from build123d import *

# Parameters (mm, degrees)
BOSS_EXTRU_1_DEPTH            = 30
ENL_V_MAT_EXTRU_1_DEPTH       = 20
BOSS_EXTRU_3_DEPTH            = 340
ENL_V_MAT_EXTRU_2_DEPTH       = 710.357976131
ENL_V_START                   = -320
ENL_V_MAT_EXTRU_5_DEPTH       = 364
R_P_TITION_CIRCULAIRE13_COUNT = 6


with BuildPart() as part:
    # Esquisse1 → Boss.-Extru.1 (new body)
    with BuildSketch(Plane(origin=(0, 0, 0), x_dir=(1, 0, 0), z_dir=(0, 1, 0))):
        Polygon((312.198829019, 291.659432373), (-96.485063179, 416.201833149), (-408.683892198, 124.542400776), (-312.198829019, -291.659432373), (96.485063179, -416.201833149), (408.683892198, -124.542400776), align=None)
    extrude(amount=BOSS_EXTRU_1_DEPTH)

    # Esquisse2 → Enlèv. mat.-Extru.1 (cut)
    with BuildSketch(Plane(origin=(0, 30, 0), x_dir=(1, 0, 0), z_dir=(0, 1, 0))):
        Polygon((403.161136898, -122.85939536), (307.979925924, 287.718088693), (-95.181210974, 410.577484053), (-403.161136898, 122.85939536), (-307.979925924, -287.718088693), (95.181210974, -410.577484053), align=None)
    extrude(amount=-ENL_V_MAT_EXTRU_1_DEPTH, mode=Mode.SUBTRACT)

    # Esquisse5 → Boss.-Extru.3 (add)
    with BuildSketch(Plane(origin=(0, 10, 0), x_dir=(1, 0, 0), z_dir=(0, 1, 0))):
        Polygon((83.204563714, -358.91453872), (43.518265641, -422.554131312), (107.157858233, -462.240429385), (146.844156306, -398.600836793), align=None)
    boss_extru_3 = extrude(amount=BOSS_EXTRU_3_DEPTH)

    # Esquisse6 → Enlèv. mat.-Extru.2 (cut, through all)
    with BuildSketch(Plane(origin=(0, 350, 0), x_dir=(1, 0, 0), z_dir=(0, 1, 0))):
        Polygon((55.305373646, -403.65272736), (96.485063179, -416.201833149), (127.942752354, -386.813728788), (146.844156306, -398.600836793), (107.157858233, -462.240429385), (43.518265641, -422.554131312), align=None)
    enl_v_mat_extru_2 = extrude(amount=-ENL_V_MAT_EXTRU_2_DEPTH, mode=Mode.SUBTRACT)

    # Esquisse7 → Enlèv. mat.-Extru.5 (cut)
    with BuildSketch(Plane(origin=(0, 350, 0), x_dir=(1, 0, 0), z_dir=(0, 1, 0)).offset(ENL_V_START)):
        Polygon((58.044458918, -399.260423737), (55.305373646, -403.65272736), (96.485063179, -416.201833149), (127.942752354, -386.813728788), (123.550448731, -384.074643516), (95.181210974, -410.577484053), align=None)
    enl_v_mat_extru_5 = extrude(amount=ENL_V_MAT_EXTRU_5_DEPTH, mode=Mode.SUBTRACT)

    # Répétition circulaire13: Boss.-Extru.3, Enlèv. mat.-Extru.2, Enlèv. mat.-Extru.5 ×6 about axis
    r_p_tition_circulaire13_axis = Axis((0, 0, 0), (0, 1, 0))
    add([boss_extru_3.rotate(r_p_tition_circulaire13_axis, i * 360 / R_P_TITION_CIRCULAIRE13_COUNT) for i in range(1, R_P_TITION_CIRCULAIRE13_COUNT)])
    add([enl_v_mat_extru_2.rotate(r_p_tition_circulaire13_axis, i * 360 / R_P_TITION_CIRCULAIRE13_COUNT) for i in range(1, R_P_TITION_CIRCULAIRE13_COUNT)], mode=Mode.SUBTRACT)
    add([enl_v_mat_extru_5.rotate(r_p_tition_circulaire13_axis, i * 360 / R_P_TITION_CIRCULAIRE13_COUNT) for i in range(1, R_P_TITION_CIRCULAIRE13_COUNT)], mode=Mode.SUBTRACT)


solid = part.part
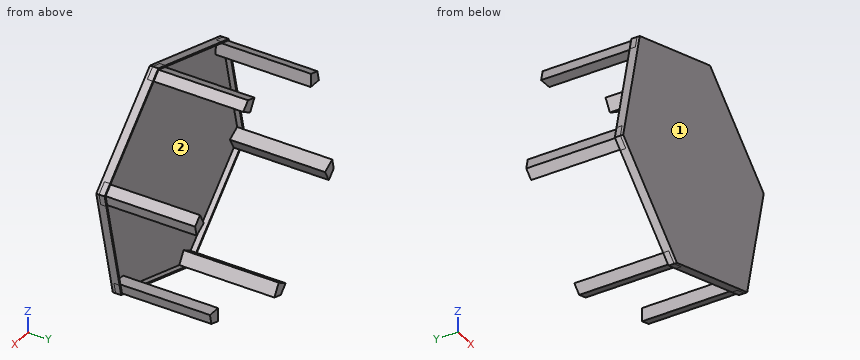
Read the model definition and answer for the solid it produces. Units are mm, in the model's axes. Face numbers are marked on the shaded views. Coordinates: 2 decimals unless noted, no trailing zeros. Write each loop counter-clockwise with the first axis right and the second up, starting at its lowest first coordinate (ties: lowest second). Pieces come first, ordered by that corner, then holes. Notation, with made-up numbers: M -11,39.5 L 30,39.5 A20 cw 30,72.5 Z; hole C 22.5,-33 d11. An arc over 180 degrees is marked long. Use a Markdown table: item, result.
Q1. Determine the mould class of the marked faces 1 and 2 for opening direction Z: released by +Z, released by -Z, zero draft, split by the parting line, or undercut.
Answer block:
| item | result |
|---|---|
| face 1 | zero draft |
| face 2 | undercut |
Q2. Each of these flat-tipped pins is pushed along its axis until it touches: pin 1 Ø2 at (x, z) = (135.5, 202.5) entering from -Y; pin 2 Ø1.5 at (x, y) = (291.5, 215.5) entering from -Z; pin 3 Ø8 at (x, y) = (76.5, 265.5) entering from +Z; pin 4 Ø4 at (x, y) = (-287, 246) entering from +Z. Where does it stop, or does it pass through?
Answer block:
| item | result |
|---|---|
| pin 1 | stops at y = 0 |
| pin 2 | stops at z = -292.97 |
| pin 3 | stops at z = 406.1 |
| pin 4 | stops at z = 294.72 |
Q3. The part is cut by section C-C, the plane x = 37. Write down the section's boundary in (y, z), then the cut area to 3 significant figures.
Answer block:
| item | result |
|---|---|
| outline | M 0,-375.52 L 30,-375.52 L 30,-370.3 L 10,-370.3 L 10,392.85 L 30,392.85 L 30,398.07 L 0,398.07 Z |
| area | 7,950 mm2 |
Q4. The part is cut by section A-A, the plane y = 203.5. Write down the section's boundary in (x, z).
Answer block:
| item | result |
|---|---|
| outline | M -403.16,-122.86 L -374.79,-149.36 L -352.43,-107.4 L -394.39,-85.04 Z; M -316.75,249.9 L -269.23,251.51 L -270.84,299.04 L -307.98,287.72 Z; M -123.55,-384.07 L -95.18,-410.58 L -58.04,-399.26 L -83.2,-358.91 Z; M 58.04,399.26 L 83.2,358.91 L 123.55,384.07 L 95.18,410.58 Z; M 269.23,-251.51 L 270.84,-299.04 L 307.98,-287.72 L 316.75,-249.9 Z; M 352.43,107.4 L 394.39,85.04 L 403.16,122.86 L 374.79,149.36 Z |
Q5. Straight lines are drawn through the part: L1, parallel to Y at x = 75.5, z = -285; L2, parallel to X at y = 28, z = 205; L3, parallel to Z at x = -366, y = 282. For each, find the intervals that lie inside material, in ascending order. Write a range as [from, to].
Answer block:
| item | result |
|---|---|
| L1 | y = [0, 10] |
| L2 | x = [-332.29, -327.16], [315.24, 322.56] |
| L3 | z = [-132.86, -100.17] |
Q6. The part is cut by section B-B, the plane x = -332.5. Write down the section's boundary in (y, z).
Answer block:
| item | result |
|---|---|
| outline | M 0,-195.71 L 30,-195.71 L 30,-188.87 L 10,-188.87 L 10,181.95 L 30,181.95 L 30,204.09 L 0,204.09 Z |
